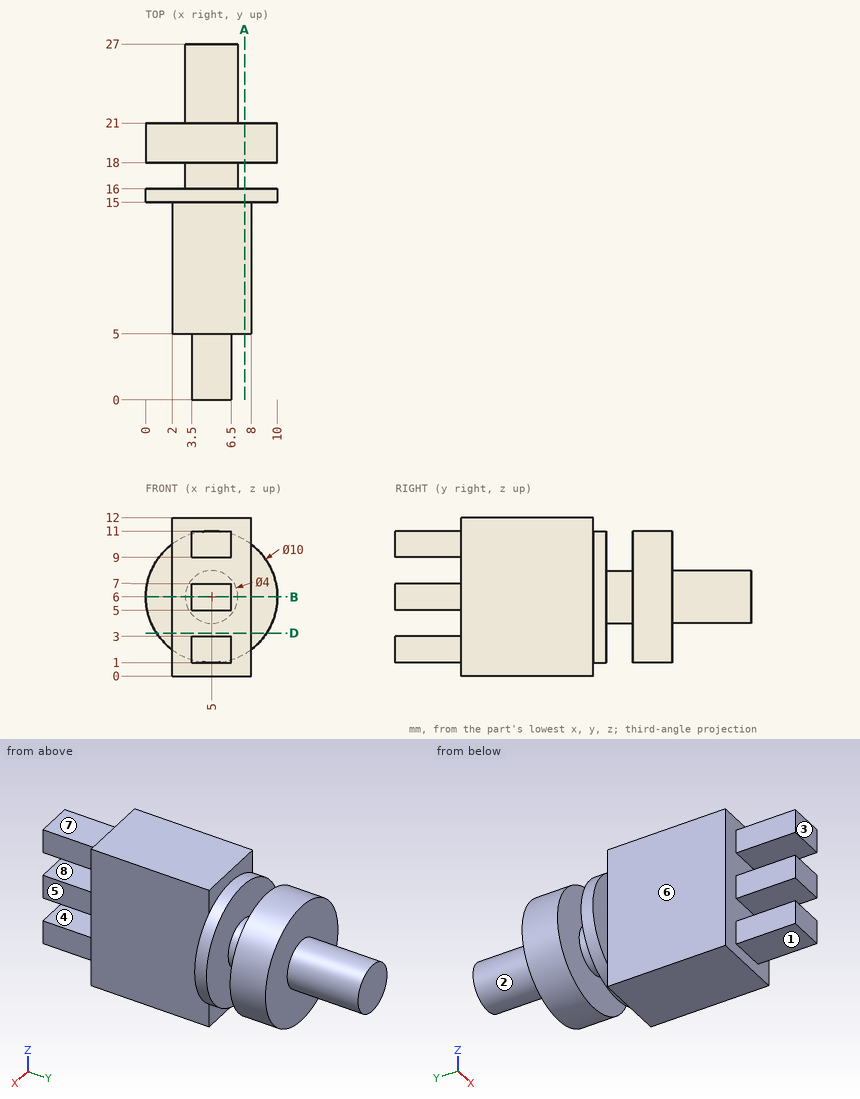
Job drawing, mm, ordinate dimensions from the low corner. One solid piece. A direction names the side the tool comes from. Give positions to 0.01 mm unless a question says otherwise; leave off trailing zeros. Order: outer loops, then holes, each group sorted by start corner. A loop starts at its lowest first (then second) coordinate and runs counter-clockwise, first axis right, second up. Notation, with made-up numbers: (67.5, 82.5) - (71.5, 82.5) arc R25 ccw to (71.5, 107.5) - close; hole circle Ø11 at (33, 77.5). An arc over 180 degrees is marked (long way). Return JSON: item names as keys, results as strings.
1) Cut at D-D, the plane z = 3.25. Give the cut face in (x, y).
Geometry says:
{"outline": "(0.82, 15) - (2, 15) - (2, 5) - (8, 5) - (8, 15) - (9.18, 15) - (9.18, 16) - (0.82, 16) - close; (0.82, 18) - (9.18, 18) - (9.18, 21) - (0.82, 21) - close"}
2) Probe line 1 (Y direction, x = 8.75, z = 3.5); line 2 (Y direction, x = 4, z = 2.5); line 3 (X direction, y = 13.5, z = 5.25). List the from-to ranges inside material, lowest first. Write a range as from..to.
Geometry says:
{"line 1": "15..16, 18..21", "line 2": "0..16, 18..21", "line 3": "2..8"}
3) Cut at B-B, the plane z = 6. Give the cut face in (x, y), plus the area to 3 significant figures.
Geometry says:
{"outline": "(0, 15) - (2, 15) - (2, 5) - (3.5, 5) - (3.5, 0) - (6.5, 0) - (6.5, 5) - (8, 5) - (8, 15) - (10, 15) - (10, 16) - (7, 16) - (7, 18) - (10, 18) - (10, 21) - (7, 21) - (7, 27) - (3, 27) - (3, 21) - (0, 21) - (0, 18) - (3, 18) - (3, 16) - (0, 16) - close", "area": "147 mm²"}
4) Cut at A-A, the plane x = 7.5. Give the cut face in (y, z), plus the area to 3 significant figures.
Geometry says:
{"outline": "(5, 0) - (15, 0) - (15, 1.67) - (16, 1.67) - (16, 10.33) - (15, 10.33) - (15, 12) - (5, 12) - close; (18, 1.67) - (21, 1.67) - (21, 10.33) - (18, 10.33) - close", "area": "155 mm²"}
5) 3-axis set-ups, long thin cutter, end or side, ignore diameter. For the marked faces 5, 6, 7 and 8: which of +Z, -Z, +X, -X, +Y, -Y reach the whole face in a straight line?
Geometry says:
{"face 5": "+Z, -Z, +X, -Y", "face 6": "+Z, -Z, -X, -Y", "face 7": "+Z, +X, -X, -Y", "face 8": "+X, -X, -Y"}
6) Pull direction Z, two halves, no side cores. Call the marked faces 1, 2, 3 and 4: pulls with the +Z half, pulls with the -Z half, needs draft (parallel to the pull), parting line crosses it, or undercut.
Geometry says:
{"face 1": "pulls with the -Z half", "face 2": "parting line crosses it", "face 3": "needs draft", "face 4": "undercut"}
7) Flat gauge pins, fed straight in: P1, Ø1.5, axis at x = 5, y = 2.5, coming from the -Z side; P2, Ø3, axis at y = 8, z = 7.5, coming from the +X side; P3, Ø1, axis at y = 10, z = 2.5, coming from the -X side; P4, Ø5, axis at x = 2.5, z = 8.5, coming from the +Y side. Where does each tip first touch, or does it go through?
Geometry says:
{"P1": "z = 1", "P2": "x = 8", "P3": "x = 2", "P4": "y = 27"}
